Part model, mm, in its own coordinate system. Face numbers are marked on the shaded views. A direction names the side the tool comes from. Give positions to 0.01 mm unless a question says otherwise; leave off trailing zeros. Write each loop counter-clockwise with the first axis right and the second up, starting at its lowest first coordinate (ties: lowest second). Pieces come first, ordered by that corner, then holes. Notation, with made-up numbers: (-2.75, -35) - (29.25, -35) arc R9 ccw to (29.25, -25) - close; hole circle Ø8 at (77.5, -1.5). An arc over 180 degrees is marked (long way). Answer in a Markdown table with one row per item. Add a question column.
1. Which spindle directions (+Z, -Z, +X, -X, +Y, -Y) get a long thin tool onto all of the face, cutting with end or side? Do the marked faces 4, 5 and 6. Say none if no direction does.
2. Band-saw the part on B-B on x = 0. Write the cut outline in (y, z), plus the area to 3 significant figures.
3. Pull direction X, two halves, no side cores. Call the marked faces 1, 2 and 3: released by +X, released by -X, zero draft, split by the parting line, or undercut.
4. Band-saw the part on C-C on y = -5. Write the cut outline in (x, z).
5. Probe line 1 along Z through (x, y) = (0, -24); line 2 along Y through (x, z) = (65.5, -28.5); line 3 along Y through (x, z) = (-4.5, -45.5). List the from-to ranges inside material, lowest first.
6. Band-saw the part on D-D on x = 112. Write the cut outline in (y, z).
7. Drop flat-ended pins along their axis: pin 1 Ø5 at (x, y) = (43.5, -61) entering from -Z; pin 2 Ø8 at (x, y) = (119.5, -9.5) entering from -Z; pin 3 Ø2 at (y, z) = (-34.5, 31.5) entering from -X. Give the stop position or say it passes through.
8. Band-saw the part on A-A on y = -60. Write the cut outline in (x, z).
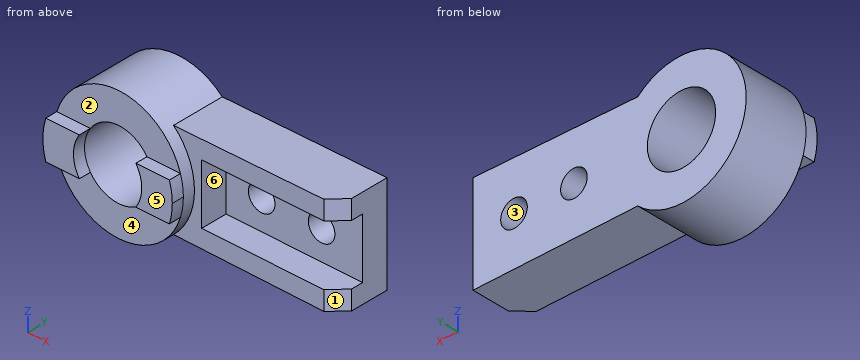
```python
from build123d import *

# Parameters (mm, degrees)
F0_R      = 54
F0_R_2    = 28.5
F1_DEPTH  = 54
F3_DEPTH  = 10
F5_DEPTH  = 44
F6_W      = 114
F6_H      = 50
F7_DEPTH  = 22
F8_SIZE   = 12
F9_R      = 11.1
F10_DEPTH = 22


# Not quite as in the source:
# - after a boolean that leaves OpenCascade's solid faulty, fix() repairs it


with BuildPart() as f1:
    # F0 (on Front) → F1 (new body)
    with BuildSketch(Plane.XZ):
        Circle(F0_R)
        Circle(F0_R_2, mode=Mode.SUBTRACT)
    extrude(amount=F1_DEPTH)

    # F2 (on face) → F3 (join)
    with BuildSketch(Plane.XZ.offset(54)):
        with BuildLine():
            Line((-23.5849528301, 16), (-51.5751878329, 16))
            ThreePointArc((-51.5751878329, 16), (-54, 0), (-51.5751878329, -16))
            Line((-51.5751878329, -16), (-23.5849528301, -16))
            ThreePointArc((-23.5849528301, -16), (-28.5, 0), (-23.5849528301, 16))
        make_face()
        with BuildLine():
            ThreePointArc((51.5751878329, -16), (53.3903556037, -8.0913489921), (54, 0))
            ThreePointArc((54, 0), (53.3903556037, 8.0913489921), (51.5751878329, 16))
            Line((51.5751878329, 16), (23.5849528301, 16))
            ThreePointArc((23.5849528301, 16), (27.2435419472, 8.368955859), (28.5, 0))
            ThreePointArc((28.5, 0), (27.2435419472, -8.368955859), (23.5849528301, -16))
            Line((23.5849528301, -16), (51.5751878329, -16))
        make_face()
    extrude(amount=F3_DEPTH)

    add(f1.part.fix(), mode=Mode.REPLACE)

    # F4 (on face) → F5 (join)
    with BuildSketch(Plane(origin=(0, 0, 0), x_dir=(-1, 0, 0), z_dir=(0, 1, 0))):
        with BuildLine():
            Line((-174, 41), (-174, 0))
            Line((-174, 0), (-174, -41))
            Line((-174, -41), (-36.5173199288, -39.7804643666))
            ThreePointArc((-36.5173199288, -39.7804643666), (-54, 0), (-36.5173199288, 39.7804643666))
            Line((-36.5173199288, 39.7804643666), (-174, 41))
        make_face()
    extrude(amount=-F5_DEPTH)

    # F6 (on face) → F7 (cut)
    with BuildSketch(Plane.XZ.offset(44)):
        with Locations((117, 0)):
            Rectangle(F6_W, F6_H)
    extrude(amount=-F7_DEPTH, mode=Mode.SUBTRACT)

    # F8
    f8_edges = [f1.edges().sort_by_distance(p)[0] for p in [
        (174, -44, 33),
        (174, -44, -33),
    ]]
    chamfer(f8_edges, length=F8_SIZE)

    # F9 (on face) → F10 (cut, through all)
    with BuildSketch(Plane.XZ.offset(22)):
        with Locations((139.781537652, 0)):
            Circle(F9_R)
        with Locations((89.781537652, 0)):
            Circle(F9_R)
    extrude(amount=-F10_DEPTH, mode=Mode.SUBTRACT)


solid = f1.part
```
Values:
| question | item | result |
|---|---|---|
| 1 | face 4 | -Z, +X, -X, -Y |
| 1 | face 5 | +Z, -Z, +X, -X, -Y |
| 1 | face 6 | +X, -Y |
| 2 | outline | (-54, -54) - (0, -54) - (0, -28.5) - (-54, -28.5) - close; (-54, 28.5) - (0, 28.5) - (0, 54) - (-54, 54) - close |
| 2 | area | 2,750 mm² |
| 3 | face 1 | released by +X |
| 3 | face 2 | zero draft |
| 3 | face 3 | undercut |
| 4 | outline | (36.52, -39.78) - (174, -41) - (174, 41) - (36.52, 39.78) arc R54 ccw (long way) to start; hole circle Ø57 at (0, 0); hole circle Ø22.2 at (89.78, 0); hole circle Ø22.2 at (139.78, 0) |
| 5 | line 1 | z = -54 to -28.5, 28.5 to 54 |
| 5 | line 2 | y = -44 to 0 |
| 5 | line 3 | y = -54 to 0 |
| 6 | outline | (-44, -40.45) - (0, -40.45) - (0, 40.45) - (-44, 40.45) - (-44, 25) - (-22, 25) - (-22, -25) - (-44, -25) - close |
| 7 | pin 1 | stops at z = -16 |
| 7 | pin 2 | stops at z = -40.55 |
| 7 | pin 3 | stops at x = -44.56 |
| 8 | outline | (-51.58, -16) - (-23.58, -16) arc R28.5 cw to (-23.58, 16) - (-51.58, 16) arc R54 ccw to start; (23.58, -16) - (51.58, -16) arc R54 ccw to (51.58, 16) - (23.58, 16) arc R28.5 cw to start |
